Here's the drawing with two shaded views (mm, measured from the low corner). I have some questions. A direction names the side the tool comes from. Coordinates: 2 decimals unless noted, no trailing zeros. Write each loop counter-clockwise with the first axis right and the second up, starting at its lowest first coordinate (ties: lowest second). Pieces come first, ordered by that corner, then holes.
Item 1: For the marked faces 4, 5 and 6, which set-ups out of +Z, -Z, +X, -X, +Y, -Y let a thin tool reach every point of the face, with its end or its side?
Item 2: If we section it at C-C (z = 0.5): Please give me the cut outline in (x, y) (3 decimals).
Item 3: If we section it at B-B (x = 15.75): Please give me the cut outline in (y, z), then the cut area to 3 significant figures.
Item 4: If I drill on line 1 (X direction, y = 2.25, z = 2.25); line 2 (Y direction, x = 15.75, z = 1.5); line 3 (Y direction, x = 12.5, z = 5.5), over which ranges is the centre line in solid material (lowest first)?
Item 5: We'd pull the mould along X, two halves only. Please class the marked faces 1, 2 and 3: +X half, -X half, draft (parallel to the pull), parting line (faces both ways), or undercut.
Item 6: If we section it at A-A (y = 19.5): Please give me the cut outline in (x, z), then the cut area to 3 significant figures.
Item 7: If we section it at D-D (x = 12): Please give me the cut outline in (y, z).
Item 8: I'm going to push flat-ended pins straight in: pin 1 Ø1.1 at (x, y) = (3.175, 3.175) entering from +Z; pin 2 Ø1.9 at (x, z) = (8, 4) entering from +Y. Where does each tip first touch, or does it pass through?
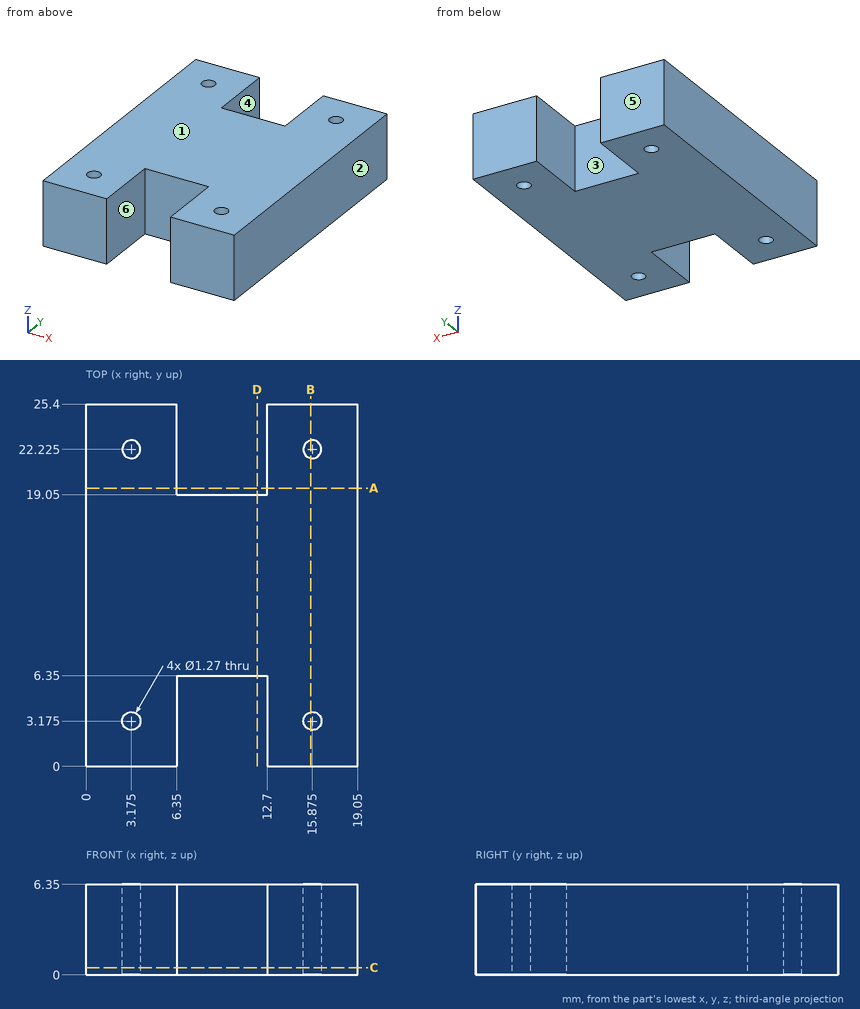
Answer list:
1. face 4: +Z, -Z, +Y
1. face 5: +Z, -Z, +X, -X, +Y
1. face 6: +Z, -Z, -Y
2. outline: (0, 0) - (6.35, 0) - (6.35, 6.35) - (12.7, 6.35) - (12.7, 0) - (19.05, 0) - (19.05, 25.4) - (12.7, 25.4) - (12.7, 19.05) - (6.35, 19.05) - (6.35, 25.4) - (0, 25.4) - close; hole circle Ø1.27 at (3.175, 3.175); hole circle Ø1.27 at (3.175, 22.225); hole circle Ø1.27 at (15.875, 3.175); hole circle Ø1.27 at (15.875, 22.225)
3. outline: (0, 0) - (2.55, 0) - (2.55, 6.35) - (0, 6.35) - close; (3.8, 0) - (21.6, 0) - (21.6, 6.35) - (3.8, 6.35) - close; (22.85, 0) - (25.4, 0) - (25.4, 6.35) - (22.85, 6.35) - close
3. area: 145 mm2
4. line 1: x = 0 to 6.35, 12.7 to 19.05
4. line 2: y = 0 to 2.55, 3.8 to 21.6, 22.85 to 25.4
4. line 3: y = 6.35 to 19.05
5. face 1: draft
5. face 2: +X half
5. face 3: undercut
6. outline: (0, 0) - (6.35, 0) - (6.35, 6.35) - (0, 6.35) - close; (12.7, 0) - (19.05, 0) - (19.05, 6.35) - (12.7, 6.35) - close
6. area: 80.6 mm2
7. outline: (6.35, 0) - (19.05, 0) - (19.05, 6.35) - (6.35, 6.35) - close
8. pin 1: passes through
8. pin 2: stops at y = 19.05
